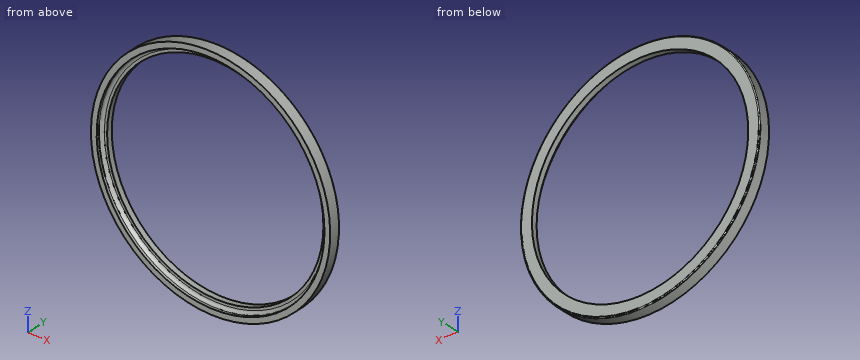
```python
from build123d import *

# Parameters (mm, degrees)
FILLET1_R = 1.5875
FILLET2_R = 0.508


with BuildPart() as part:
    # Sketch1 → Revolve1 (revolve)
    with BuildSketch(Plane.XY, mode=Mode.PRIVATE) as revolve1_sk:
        Polygon((-57.56402, 0), (-63.66002, 0), (-63.66002, -6.096), (-60.61202, -6.096), (-60.61202, -3.048), (-57.56402, -3.048), align=None)
    revolve(revolve1_sk.sketch.rotate(Axis((0, 0, 0), (0, 1, 0)), 270), axis=Axis((0, 0, 0), (0, 1, 0)))

    # Fillet1
    fillet1_edges = [part.edges().sort_by_distance(p)[0] for p in [
        (0, -3.048, 60.61202),
    ]]
    fillet(fillet1_edges, radius=FILLET1_R)

    # Fillet2
    fillet2_edges = [part.edges().sort_by_distance(p)[0] for p in [
        (0, 0, 63.66002),
    ]]
    fillet(fillet2_edges, radius=FILLET2_R)


solid = part.part
```
The listing builds one solid part. Answer for the finished solid, in the listing's coordinates (mm). Give positions to 0.01 mm unless a question says otherwise; leave off trailing zeros. Write each loop counter-clockwise with the first axis right and the second up, starting at its lowest first coordinate (ties: lowest second). Pieces come first, ordered by that corner, then holes. Notation, with made-up numbers: (-14, 80.25) -> (14, 80.25) arc R21 ccw to (14, 94.25) -> close; hole circle Ø4 at (43, 79). An arc over 180 degrees is marked (long way). Use one line per item in the form item = value.
1) Straight lines are drawn through the part: probe 1 along X at (y, z) = (-1.15, 0); probe 2 along X at (y, z) = (-5.6, 0); probe 3 along Z at (x, y) = (44, -4.5). For each, find the intervals that lie inside material, in ascending order.
Result:
probe_1 = -63.66 to -57.56, 57.56 to 63.66
probe_2 = -63.66 to -60.61, 60.61 to 63.66
probe_3 = -46.01 to -41.68, 41.68 to 46.01
2) Section A-A on x = 0 is taken. Write down the section's boundary in (y, z) (1 decimal).
Result:
outline = (-6.1, -63.7) -> (-0.5, -63.7) arc R0.5 ccw to (0, -63.2) -> (0, -57.6) -> (-3, -57.6) -> (-3, -59) arc R1.6 cw to (-4.6, -60.6) -> (-6.1, -60.6) -> close; (-6.1, 60.6) -> (-4.6, 60.6) arc R1.6 cw to (-3, 59) -> (-3, 57.6) -> (0, 57.6) -> (0, 63.2) arc R0.5 ccw to (-0.5, 63.7) -> (-6.1, 63.7) -> close
3) Section B-B on z = 0 is taken. Write down the section's boundary in (x, y) (1 decimal), plus the area to 3 significant figures.
Result:
outline = (-63.7, -6.1) -> (-60.6, -6.1) -> (-60.6, -4.6) arc R1.6 cw to (-59, -3) -> (-57.6, -3) -> (-57.6, 0) -> (-63.2, 0) arc R0.5 ccw to (-63.7, -0.5) -> close; (57.6, -3) -> (59, -3) arc R1.6 cw to (60.6, -4.6) -> (60.6, -6.1) -> (63.7, -6.1) -> (63.7, -0.5) arc R0.5 ccw to (63.2, 0) -> (57.6, 0) -> close
area = 56.7 mm²
4) Each of these flat-tipped pins is pushed along its axis until it touches: P1, Ø1, axis at y = -1, z = -32, coming from the +X side; P2, Ø2, axis at y = -1, z = 47, coming from the -X side. Where does it stop, or does it pass through?
Result:
P1 = 55.32
P2 = -44.01
